Verification items for the finished model (mm, model axes). Round coordinates to 2 decimals unless told otherwise and drop trailing zeros. Order: outer loops, then holes, each group sorted by start corner. A loop starts at its lowest first (then second) coordinate and runs counter-clockwise, first axis right, second up. Notation, with made-up numbers: M -19.75,63.5 L 38.25,63.5 A10 cw 38.25,81.5 Z; hole C 86,-26.5 d9. An arc over 180 degrees is marked long. One line per item, written item: value. Start each with the question number.
from build123d import *

# Parameters (mm, degrees)
F0_R     = 50
F1_DEPTH = 25
F2_R     = 5
F3_DEPTH = 74


with BuildPart() as f1:
    # F0 (on Front) → F1 (new body, symmetric)
    with BuildSketch(Plane.XZ):
        Circle(F0_R)
    extrude(amount=F1_DEPTH, both=True)

    # F2 (on face) → F3 (cut)
    with BuildSketch(Plane.XZ.offset(25)):
        with BuildLine():
            ThreePointArc((-19.485572, 11.25), (-18.986069, 12.455905), (-18.815699, 13.75))
            ThreePointArc((-18.815699, 13.75), (-22.521603, 18.579629), (-28.145826, 16.25))
            Line((-28.145826, 16.25), (-19.485572, 11.25))
        make_face()
        with BuildLine():
            ThreePointArc((28.145826, 16.25), (21.315699, 18.080127), (19.485572, 11.25))
            Line((19.485572, 11.25), (28.145826, 16.25))
        make_face()
        with BuildLine():
            Line((28.145826, 16.25), (19.485572, 11.25))
            ThreePointArc((19.485572, 11.25), (25.109794, 8.920371), (28.815699, 13.75))
            ThreePointArc((28.815699, 13.75), (28.645328, 15.044095), (28.145826, 16.25))
        make_face()
        with BuildLine():
            Line((-19.485572, 11.25), (-28.145826, 16.25))
            ThreePointArc((-28.145826, 16.25), (-26.315699, 9.419873), (-19.485572, 11.25))
        make_face()
        with Locations((0, -27.5)):
            Circle(F2_R)
    extrude(amount=-F3_DEPTH, mode=Mode.SUBTRACT)


solid = f1.part
1. Section check D-D (z = -40). Record the cut outline in (x, y).
2. Section check B-B (y = -11.5). Record the cut outline in (x, z).
3. Depth check by flat-ended pin: pin 1 (1.5 mm diameter, centred on x = 12, y = 1.5, fed in from -Z); pin 2 (10 mm diameter, centred on y = -7.5, z = 12.5, fed in from +X); pin 3 (1.5 mm diameter, centred on x = 37.5, y = 14.5, fed in from -Z). Enter the tip coordinate at first touch or a pass-through.
4. Draft check along Z on faces 1 (the face through (-1, 25, 1)), 2 (the face through (47.69, -0.35, 15.02)), 3 (the face through (-19, -0.4, 12.4)). Enter one of: released by +Z, released by -Z, zero draft, split by the parting line, or undercut.
5. Scan lines: line 1 along Z through (x, y) = (0, 7); line 2 along X through (y, z) = (-14, -27); line 3 along Z through (x, y) = (20, 0). Record each from-to range of solid material in increasing order.
6. Section check C-C (z = -27.5). Record the cut outline in (x, y).
7. Section check A-A (x = 0). Record the cut outline in (y, z), and give its area (3 significant figures).
Geometry check:
1. outline: M -30,-25 L 30,-25 L 30,25 L -30,25 Z
2. outline: C 0,0 d100; hole M -19.49,11.25 A5 ccw -18.82,13.75 A5 ccw long Z; hole C 0,-27.5 d10; hole M 28.15,16.25 A5 ccw long 28.82,13.75 A5 ccw Z
3. pin 1: stops at z = -48.72
3. pin 2: stops at x = 49.43
3. pin 3: stops at z = -33.9
4. face 1: zero draft
4. face 2: split by the parting line
4. face 3: undercut
5. line 1: z = -50 to -32.5, -22.5 to 50
5. line 2: x = -42.08 to -4.97, 4.97 to 42.08
5. line 3: z = -45.83 to 10.52, 16.98 to 45.83
6. outline: M -41.76,-25 L -5,-25 L -5,25 L -41.76,25 Z; M 5,-25 L 41.76,-25 L 41.76,25 L 5,25 Z
7. outline: M -25,-50 L 25,-50 L 25,-32.5 L -25,-32.5 Z; M -25,-22.5 L 25,-22.5 L 25,50 L -25,50 Z
7. area: 4,500 mm²
